Work out the finished part from the listing and answer in its coordinate system (mm). Face numbers are marked on the shaded views. A direction names the side the tool comes from. Coordinates: 2 decimals unless noted, no trailing zeros. Loops run counter-clockwise (first coordinate to the right, second up) from the corner with the lowest first, then second, coordinate; pieces in that order, holes last. Notation, with made-up numbers: (55.5, 21.5) -> (107.5, 21.5) arc R18 cw to (107.5, 43.5) -> close; hole circle Ø8 at (-25.75, 6.25). An arc over 180 degrees is marked (long way). One line per question, with ' | ' between items.
```python
from build123d import *

# Parameters (mm, degrees)
SKETCH1_R           = 7.5
BOSS_EXTRUDE1_DEPTH = 12
SKETCH3_R           = 3.425
CUT_EXTRUDE1_DEPTH  = 23.0000001
FILLET1_R           = 2.54
SKETCH4_R           = 5.08
CUT_EXTRUDE2_DEPTH  = 18.000000194
SKETCH5_W           = 44.45
SKETCH5_H           = 24
SKETCH5_R           = 3.425
BOSS_EXTRUDE2_DEPTH = 16


with BuildPart() as part:
    # Sketch1 → Boss-Extrude1 (new body, symmetric)
    with BuildSketch(Plane.XY):
        with BuildLine():
            Line((22.225, -10), (-22.225, -10))
            Line((-22.225, -10), (-22.225, -5))
            add(Edge.make_bspline(
                [(-22.225, -5), (-16.631079064, -4.98201906), (-12.322747723, -1.728386223), (-12.530535341, 3.440374129), (-9.467504716, 7.373354356)],
                knots=[0, 0, 0, 0, 0.501954987, 1, 1, 1, 1], degree=3))
            ThreePointArc((-9.467504716, 7.373354356), (0, 12), (9.467504716, 7.373354356))
            add(Edge.make_bspline(
                [(22.225, -5), (16.631079064, -4.98201906), (12.322747723, -1.728386223), (12.530535341, 3.440374129), (9.467504716, 7.373354356)],
                knots=[0, 0, 0, 0, 0.501954987, 1, 1, 1, 1], degree=3))
            Line((22.225, -5), (22.225, -10))
        make_face()
        Circle(SKETCH1_R, mode=Mode.SUBTRACT)
    extrude(amount=BOSS_EXTRUDE1_DEPTH, both=True)

    # Sketch3 → Cut-Extrude1 (cut, through all)
    with BuildSketch(Plane.XZ.offset(10)):
        with Locations((-12.7, 0)):
            Circle(SKETCH3_R)
        with Locations((12.7, 0)):
            Circle(SKETCH3_R)
    extrude(amount=-CUT_EXTRUDE1_DEPTH, mode=Mode.SUBTRACT)

    # Fillet1
    fillet1_edges = [part.edges().sort_by_distance(p)[0] for p in [
        (22.225, -5, -6),
        (-22.225, -5, 6),
    ]]
    fillet(fillet1_edges, radius=FILLET1_R)

    # Sketch4 → Cut-Extrude2 (cut, through all)
    with BuildSketch(Plane(origin=(0, -5.000000094, 0), x_dir=(-1, 0, 0), z_dir=(0, -1, 0))):
        with Locations((12.7, 0)):
            Circle(SKETCH4_R)
        with Locations((-12.7, 0)):
            Circle(SKETCH4_R)
    extrude(amount=-CUT_EXTRUDE2_DEPTH, mode=Mode.SUBTRACT)

    # Sketch5 → Boss-Extrude2 (add)
    with BuildSketch(Plane.XZ.offset(10)):
        Rectangle(SKETCH5_W, SKETCH5_H)
        with Locations((12.7, 0)):
            Circle(SKETCH5_R, mode=Mode.SUBTRACT)
        with Locations((-12.7, 0)):
            Circle(SKETCH5_R, mode=Mode.SUBTRACT)
    extrude(amount=BOSS_EXTRUDE2_DEPTH)


solid = part.part
```
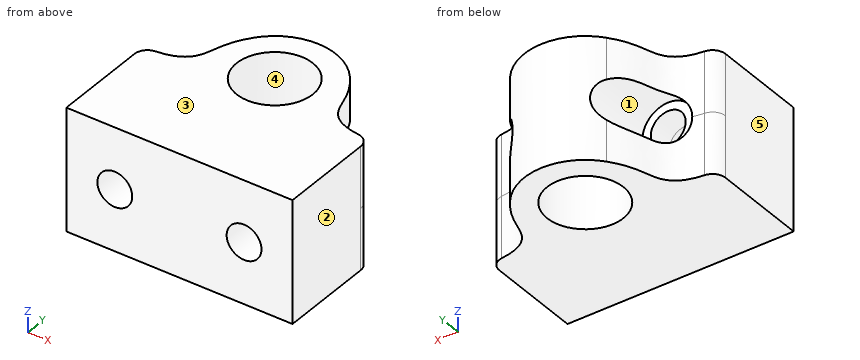
1) Find the intervals of material crossed by line 1 along Z through (x, y) = (-12.7, -7.6) (3 decimals); line 2 along X through (y, z) = (-6, -1); line 3 along Y through (x, z) = (1.5, -5.5), in increasing order.
Check values:
line 1: z = -12 to -3.425, 3.425 to 12 | line 2: x = -21.79 to -15.98, -9.42 to -4.5, 4.5 to 9.42, 15.98 to 21.79 | line 3: y = -26 to -7.35, 7.35 to 11.91
2) For the marked faces 1 and 2, determine the directions among +Z, -Z, +X, -X, +Y, -Y from which every point of the face is accessible in a straight line to the end or side of a thin tool.
Check values:
face 1: +Y | face 2: +Z, -Z, +X, +Y, -Y
3) The mould has two halves that part along X. Classify the marked faces 3, 4 and 5: released by +X, released by -X, zero draft, split by the parting line, or undercut.
Check values:
face 3: zero draft | face 4: undercut | face 5: released by -X
4) Find section A-A (x = 0). Write down the section's boundary in (y, z).
Check values:
outline: (-26, -12) -> (-7.5, -12) -> (-7.5, 12) -> (-26, 12) -> close; (7.5, -12) -> (12, -12) -> (12, 12) -> (7.5, 12) -> close
5) Find section B-B (y = -17). Write down the section's boundary in (x, z) (3 decimals).
Check values:
outline: (-22.225, -12) -> (22.225, -12) -> (22.225, 12) -> (-22.225, 12) -> close; hole circle Ø6.85 at (-12.7, 0); hole circle Ø6.85 at (12.7, 0)
6) Flat-ended cylindrical pins translate along their axes: pin 1 (12 mm diameter, centred on x = 0, y = 0, fed in from -Z); pin 2 (9 mm diameter, centred on x = 12.7, z = 0, fed in from +Y); pin 3 (8 mm diameter, centred on y = 8, z = -7.5, fed in from -X); pin 4 (8 mm diameter, centred on x = 11.5, z = 1, fed in from +Y). Find the tip coordinate at first contact, or state that the pin passes through.
Check values:
pin 1: passes through | pin 2: stops at y = -5 | pin 3: stops at x = -11.57 | pin 4: stops at y = 9.37
